Geometry: final body of the model. Coordinates: model frame, mm. A direction names the side the tool comes from. Coordinates: 2 decimals unless noted, no trailing zeros. Loops run counter-clockwise (first coordinate to the right, second up) from the corner with the lowest first, then second, coordinate; pieces in that order, holes last. Notation, with made-up numbers: (-37, 34.5) -> (-7, 34.5) arc R4 ccw to (-7, 38.5) -> close; hole circle Ø8 at (27, -17). An arc over 180 degrees is marked (long way). One line per item, written item: value. Start each with the question number.
Item 1: Ray query, probe 1 along X at (y, z) = (59, 249); probe 2 along Y at (x, z) = (41, 591.5); probe 3 along Z at (x, y) = (165.5, 72.5). Return the intervals inside material, ascending. Write a range as from..to.
Item 2: Mould query, pull axis Y, two halves, no side actions, for faces 1 (the flat face through (25.4, 55, 326)), 2 (the cylindrical face through (86.29, 51.26, 12.52)), 3 (the flat face through (95, 110.591, 339)). Classes: +Y half, -Y half, draft (parallel to the pull), parting line (faces both ways), or undercut.
Item 3: Section query C-C on y = 62.5. Return loops of the section in (x, z).
Item 4: Section query A-A on x = 100. Return loops of the section in (y, z).
Item 5: Section query D-D on x = 36. Return loops of the section in (y, z), then the cut area to 3 significant figures.
Item 6: Set-up query: faces 4 (the flat face through (95, 135.991, 313)), 5 (the cylindrical face through (94.89, 102.95, 32.64)). Return all of +Z, -Z, +X, -X, +Y, -Y with unobstructed straight access to the full face (end or side cutting, diameter ignored); none if empty.
Item 7: Section query B-B on z = 424.5. Return loops of the section in (x, y), then the cut area to 3 significant figures.
Item 8: Contact query for flat-ended pins moving along their axis: pin 1 Ø4 at (x, y) = (159, 72) entering from +Z; pin 2 Ø2 at (x, z) = (108, 346.5) entering from -Y; pin 3 Ø5 at (x, y) = (117, 92.5) entering from +Z. Output: stop coordinate, or through.
from build123d import *

# Parameters (mm, degrees)
F0_W        = 191.7510181665
F0_H        = 135.9910964966
F1_DEPTH    = 635
F2_T        = -25.4
F4_D        = 25.4
F5_R        = 25.4
F6_T1_DEPTH = 286.6829915773
F6_T3_DEPTH = 286.6829915773


# Not quite as in the source:
# - a fillet or chamfer that OpenCascade refuses, or shapes differently, is made with other operations: its cross-section is extruded or revolved along the edge and cut away or added


with BuildPart() as f1:
    # F0 (on Top) → F1 (new body)
    with BuildSketch(Plane.XY):
        with Locations((95.8755090833, 67.9955482483)):
            Rectangle(F0_W, F0_H)
    extrude(amount=F1_DEPTH)

    # F2
    f2_openings = [f1.faces().sort_by_distance(p)[0] for p in [
        (95.875509, 0, 317.5),
        (95.875509, 67.995548, 635),
    ]]
    offset(amount=F2_T, openings=f2_openings)

    # F4 (through all)
    with Locations(Plane.XY.offset(25.4)):
        with Locations((98.0245098472, 56.1208538711)):
            Hole(F4_D / 2)

    # F5
    f5_edges = [f1.edges().sort_by_distance(p)[0] for p in [
        (95.875509, 110.591096, 25.4),
    ]]
    fillet(f5_edges, radius=F5_R)

    # F6: chamfer of 50.8 on 3 edges, made by hand

    # F6_s2 → F6_t1 (cut)
    with BuildSketch(Plane.YZ.offset(-130.6414957887)):
        Polygon((0, 584.2), (50.8, 635), (0, 635), align=None)
    extrude(amount=F6_T1_DEPTH, mode=Mode.SUBTRACT)

    # F6_s4 → F6_t3 (cut)
    with BuildSketch(Plane.YZ.offset(35.7095223779)):
        Polygon((0, 584.2), (50.8, 635), (0, 635), align=None)
    extrude(amount=F6_T3_DEPTH, mode=Mode.SUBTRACT)


solid = f1.part
Reply:
1. probe 1: x = 0..25.4, 166.35..191.75
1. probe 2: y = 110.59..135.99
1. probe 3: z = 0..25.4
2. face 1: draft
2. face 2: undercut
2. face 3: -Y half
3. outline: (0, 0) -> (87.04, 0) -> (87.04, 25.4) -> (25.4, 25.4) -> (25.4, 635) -> (0, 635) -> close; (109.01, 0) -> (191.75, 0) -> (191.75, 635) -> (166.35, 635) -> (166.35, 25.4) -> (109.01, 25.4) -> close
4. outline: (0, 0) -> (43.58, 0) -> (43.58, 25.4) -> (0, 25.4) -> close; (68.67, 0) -> (135.99, 0) -> (135.99, 635) -> (110.59, 635) -> (110.59, 50.8) arc R25.4 cw to (85.19, 25.4) -> (68.67, 25.4) -> close
5. outline: (0, 0) -> (135.99, 0) -> (135.99, 635) -> (110.59, 635) -> (110.59, 50.8) arc R25.4 cw to (85.19, 25.4) -> (0, 25.4) -> close
5. area: 19,100 mm²
6. face 4: +Z, -Z, +X, -X, +Y
6. face 5: +Z, -Y
7. outline: (0, 0) -> (25.4, 0) -> (25.4, 110.59) -> (166.35, 110.59) -> (166.35, 0) -> (191.75, 0) -> (191.75, 135.99) -> (0, 135.99) -> close
7. area: 10,500 mm²
8. pin 1: stops at z = 25.4
8. pin 2: stops at y = 110.59
8. pin 3: stops at z = 27.37
